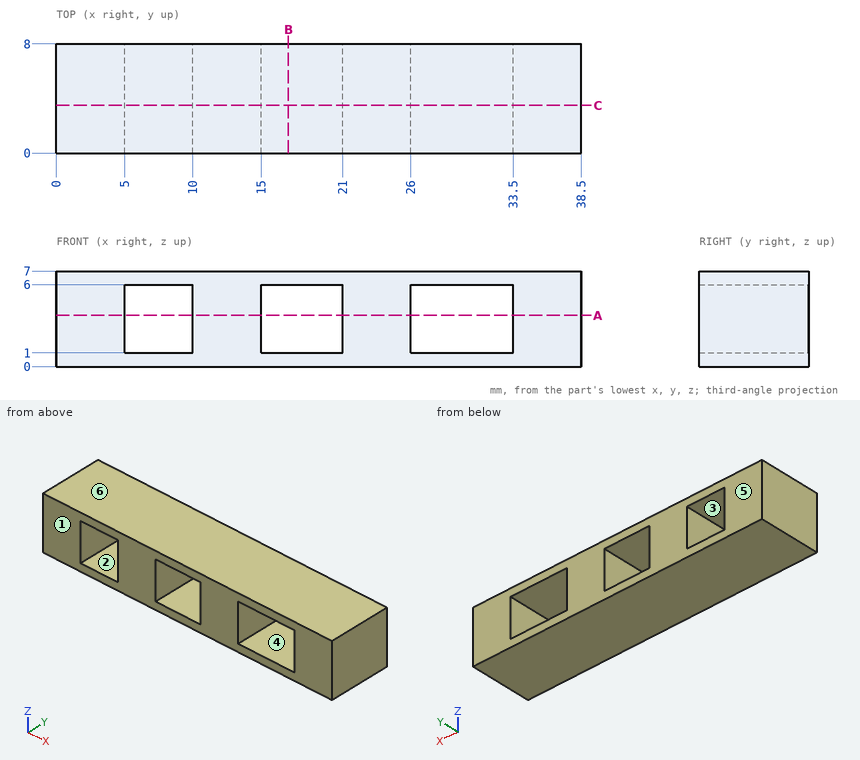
Here's the drawing with two shaded views (mm, measured from the low corner). I have some questions. A direction names the side the tool comes from. Coordinates: 2 decimals unless noted, no trailing zeros. Write each loop counter-clockwise with the first axis right and the second up, starting at its lowest first coordinate (ties: lowest second). Pieces come first, ordered by that corner, then holes.
Item 1: I want a section at A-A on z = 3.75. Write out the boundary of the cut face in (x, y), and give its area (3 significant figures).
Item 2: I want a section at B-B on x = 17. Write out the boundary of the cut face in (y, z).
Item 3: On a 3-axis mill with a long thin cutter (end or side, diameter ignored), from which of +Z, -Z, +X, -X, +Y, -Y can I reach the whole of each face in a straight line? I mean the marked faces 1 and 2. Say none if no direction works.
Item 4: If I drill on line 1 (X direction, y = 1.5, z = 4.75); line 2 (Z direction, x = 29, y = 3), over which ranges is the centre line in solid material (lowest first)?
Item 5: I want a section at C-C on y = 3.5. Write out the boundary of the cut face in (x, z), and give its area (3 significant figures).
Item 6: If we mould it in two halves opening along Z, with no side actions, what happens to the marked faces 3, 4, 5 and 6? For each: +Z half, -Z half, draft (parallel to the pull), parting line (faces both ways), or undercut.
Findings below:
1. outline: (0, 0) - (5, 0) - (5, 8) - (0, 8) - close; (10, 0) - (15, 0) - (15, 8) - (10, 8) - close; (21, 0) - (26, 0) - (26, 8) - (21, 8) - close; (33.5, 0) - (38.5, 0) - (38.5, 8) - (33.5, 8) - close
1. area: 160 mm2
2. outline: (0, 0) - (8, 0) - (8, 1) - (0, 1) - close; (0, 6) - (8, 6) - (8, 7) - (0, 7) - close
3. face 1: +Z, -Z, +X, -X, -Y
3. face 2: +Y, -Y
4. line 1: x = 0 to 5, 10 to 15, 21 to 26, 33.5 to 38.5
4. line 2: z = 0 to 1, 6 to 7
5. outline: (0, 0) - (38.5, 0) - (38.5, 7) - (0, 7) - close; hole (5, 1) - (10, 1) - (10, 6) - (5, 6) - close; hole (15, 1) - (21, 1) - (21, 6) - (15, 6) - close; hole (26, 1) - (33.5, 1) - (33.5, 6) - (26, 6) - close
5. area: 177 mm2
6. face 3: undercut
6. face 4: undercut
6. face 5: draft
6. face 6: +Z half
